Print and shaded views of the part. All mm, measured from the part's lowest x, y and z. Give positions to 0.01 mm unless a question says otherwise; leave off trailing zeros. Loops run counter-clockwise (first coordinate to the right, second up) from the corner with the lowest first, then second, coordinate; pieces in that order, holes last.
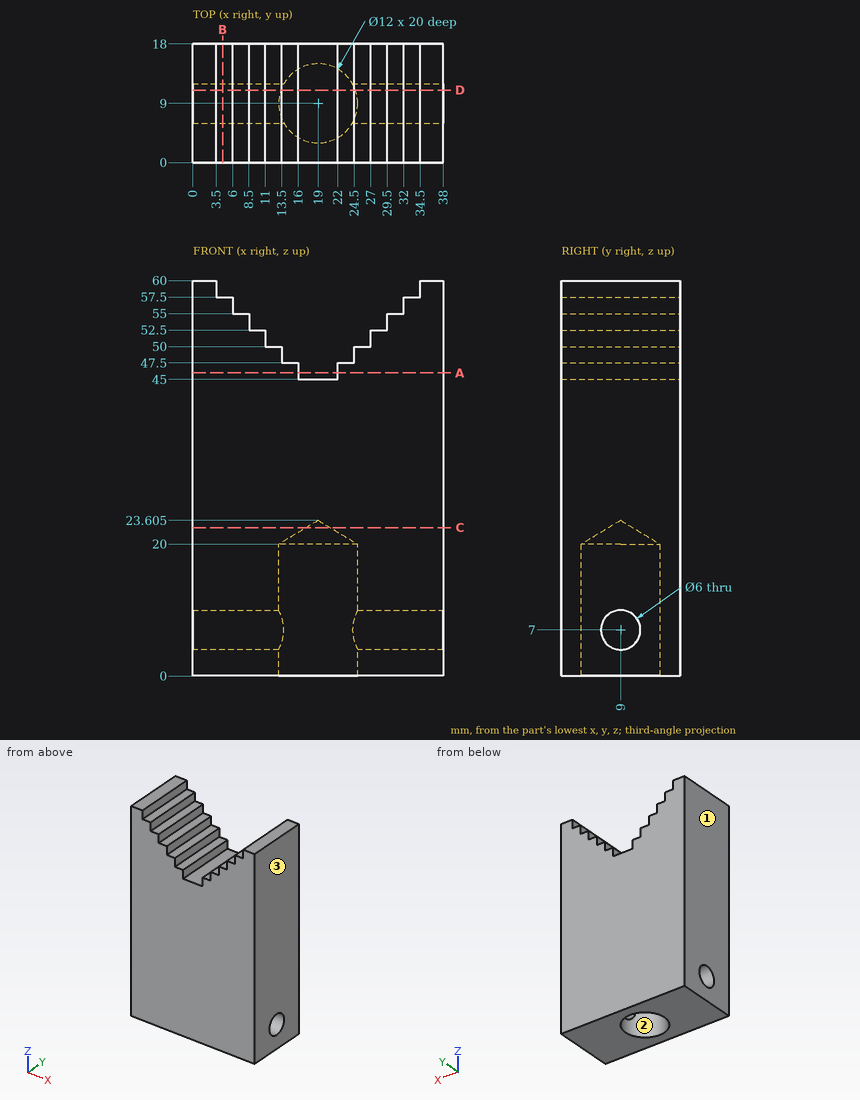
1. Saw through at D-D, the plane y = 11. Count the separate pieces of the cut face and the enclosed holes in it, and give its area (3 significant figures).
Responses:
separate pieces: 3
enclosed holes: 0
area: 1,640 mm2
2. Probe line 1 along X through (y, z) = (8.5, 52); line 2 along Z through (x, y) = (10.5, 9); line 3 along Y through (x, z) = (4, 7). List the from-to ranges inside material, lowest first.
Responses:
line 1: x = 0 to 11, 27 to 38
line 2: z = 0 to 4, 10 to 52.5
line 3: y = 0 to 6, 12 to 18
3. Pull direction X, two halves, no side cores. Call the marked faces 1, 2 and 3: released by +X, released by -X, zero draft, split by the parting line, or undercut.
Responses:
face 1: released by -X
face 2: undercut
face 3: released by +X
4. Saw through at C-C, the plane z = 22.5. List the corners of the cut face in (x, y), and give its area (3 significant figures).
Responses:
outline: (0, 0) - (38, 0) - (38, 18) - (0, 18) - close; hole circle Ø3.68 at (19, 9)
area: 673 mm2
5. Drop flat-ended pins along their axis: pin 1 (6 mm diameter, centred on x = 22.5, y = 13, fed in from +Z); pin 2 (1 mm diameter, centred on x = 18.5, y = 10, fed in from -Z); pin 3 (7 mm diameter, centred on x = 19, y = 9, fed in from -Z). Give the stop position or say it passes through.
Responses:
pin 1: stops at z = 50
pin 2: stops at z = 22.63
pin 3: stops at z = 21.5
6. Saw through at A-A, the plane z = 46. List the corners of the cut face in (x, y).
Responses:
outline: (0, 0) - (16, 0) - (16, 18) - (0, 18) - close; (22, 0) - (38, 0) - (38, 18) - (22, 18) - close
7. Saw through at B-B, the plane x = 4.5. List the corners of the cut face in (y, z).
Responses:
outline: (0, 0) - (18, 0) - (18, 57.5) - (0, 57.5) - close; hole circle Ø6 at (9, 7)
